from build123d import *

# Parameters (mm, degrees)
PAD_DEPTH    = 17
PAD001_DEPTH = 2
PAD002_DEPTH = 1.8
SKETCH003_W  = 32
SKETCH003_H  = 11
PAD003_DEPTH = 5
SKETCH004_W  = 3.1
SKETCH004_H  = 3.1
POCKET_DEPTH = 3.1
FILLET_R     = 3
FILLET001_R  = 1


with BuildPart() as part:
    # Sketch → Pad (new body)
    with BuildSketch(Plane.XY):
        with BuildLine():
            Line((-10, 0), (-10, 5))
            Line((-10, 5), (5, 5))
            Line((5, 5), (5, -10))
            Line((5, -10), (0, -10))
            Line((0, -7.05), (0, -10))
            Line((0, -7.05), (0.143534, -7.05))
            ThreePointArc((0.143534, -7.05), (3.05, -6.3), (0.143534, -5.55))
            Line((0, -5.55), (0.143534, -5.55))
            Line((0, 0), (0, -5.55))
            Line((0, 0), (-5.55, 0))
            Line((-5.55, 0), (-5.55, 0.143534))
            ThreePointArc((-5.55, 0.143534), (-6.3, 3.05), (-7.05, 0.143534))
            Line((-7.05, 0), (-7.05, 0.143534))
            Line((-10, 0), (-7.05, 0))
        make_face()
    extrude(amount=-PAD_DEPTH)

    # Sketch001 (on Face16 of Pad) → Pad001 (join)
    with BuildSketch(Plane(origin=(0, 0, -17), x_dir=(1, 0, 0), z_dir=(0, 0, -1))):
        Polygon((5, -5), (-10, -5), (-10, 0), (0, 10), (5, 10), align=None)
    extrude(amount=PAD001_DEPTH)

    # Sketch002 (on Face1 of Pad001) → Pad002 (join)
    with BuildSketch(Plane.XY):
        Polygon((0, -10), (0, 0), (-10, 0), align=None)
    extrude(amount=-PAD002_DEPTH)

    # Sketch003 (on Face10 of Pad002) → Pad003 (join)
    with BuildSketch(Plane.XZ):
        with Locations((-26, -13.5)):
            Rectangle(SKETCH003_W, SKETCH003_H)
    extrude(amount=-PAD003_DEPTH)

    # Sketch004 (on Face22 of Pad003) → Pocket (cut)
    with BuildSketch(Plane.XZ):
        with Locations((-36.45, -13.45)):
            Rectangle(SKETCH004_W, SKETCH004_H)
    extrude(amount=-POCKET_DEPTH, mode=Mode.SUBTRACT)

    # Fillet
    fillet_edges = [part.edges().sort_by_distance(p)[0] for p in [
        (-10, 2.5, -8),
        (-42, 2.5, -8),
        (-42, 2.5, -19),
        (-10, 0, -18),
    ]]
    fillet(fillet_edges, radius=FILLET_R)

    # Fillet001
    fillet001_edges = [part.edges().sort_by_distance(p)[0] for p in [
        (-10, 5, -2.5),
        (-10.87868, 5, -7.12132),
        (-2.5, 5, 0),
        (-26, 5, -8),
        (5, 5, -9.5),
        (-41.12132, 5, -8.87868),
        (-17, 5, -19),
        (-42, 5, -13.5),
        (-41.12132, 5, -18.12132),
        (5, -2.5, 0),
        (5, -10, -9.5),
        (5, -2.5, -19),
        (0, 0, -9.4),
    ]]
    fillet(fillet001_edges, radius=FILLET001_R)


solid = part.part
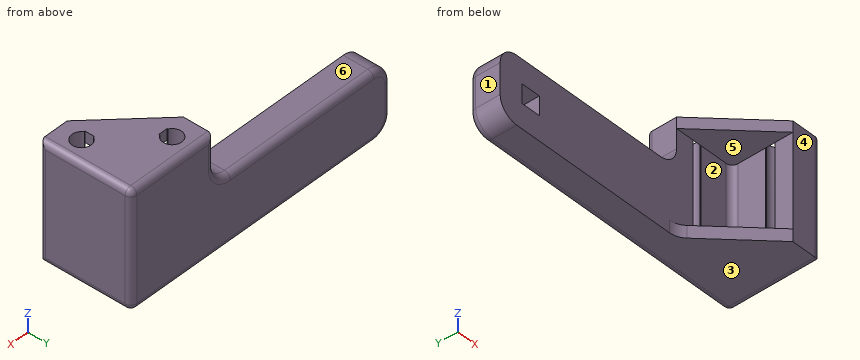
Design review of the part built by this model. Coordinates are the model's own, in mm. Face numbers are marked on the shaded views. A direction names the side the tool comes from. Round coordinates to 2 decimals unless told otherwise and drop trailing zeros. Loops run counter-clockwise (first coordinate to the right, second up) from the corner with the lowest first, then second, coordinate; pieces in that order, holes last. Notation, with made-up numbers: (20, 58) - (51, 58) arc R13 cw to (51, 82) - close; hole circle Ø8 at (52.25, -10). An arc over 180 degrees is marked (long way). One line per item, written item: value. Start each with the question number.
1) Consider section C-C on y = -4. Give the boundary of the cut face in (x, z), then the cut area to 3 significant figures.
2) Insertion check: pin 1 Ø1.5 at (x, y) = (-36.5, 2.5) entering from +Z; pin 2 Ø1.4 at (x, z) = (-3, -6.5) entering from -Y; pin 3 Ø0.9 at (y, z) = (-8.5, -10.5) entering from -X. Each pin has a flat end and moves straight along its axis. Give the tip position at first contact, or say it passes through.
3) Consider section A-A on y = 1.5. Give the boundary of the cut face in (x, z), then the cut area to 3 significant figures.
4) Draft analysis for pull direction Z (two halves, no side actions). For the marked faces 1, 2 and 3, state which applies: +Z half, -Z half, draft (parallel to the pull), parting line (faces both ways), or undercut.
5) For the marked faces 4, 5 and 6, list the 3-axis set-ups (+Z, -Z, +X, -X, +Y, -Y) from which the entire face can be reached by the end or side of a thin tool; tool diameter is ignored.
6) To check wall thickness, follow L1, parallel to X at y = -6.3, z = -10; L2, parallel to Y at x = 1.5, z = -6.5; L3, parallel to Z at x = -4.5, y = -3.5. State the ranges of each line that lie inside material, in increasing order. Write a range as from..to.
7) Consider section D-D on z = -13.25. Give the boundary of the cut face in (x, y).
8) Consider section B-B on x = -6.3. Give the boundary of the cut face in (y, z).
Reported:
1. outline: (-6, -19) - (4, -19) arc R1 ccw to (5, -18) - (5, -1) arc R1 ccw to (4, 0) - (-6, 0) - (-6, -1.8) - (0, -1.8) - (0, -17) - (-6, -17) - close
1. area: 117 mm^2
2. pin 1: stops at z = -8
2. pin 2: stops at y = 0
2. pin 3: stops at x = 0
3. outline: (-42, -16) arc R3 ccw to (-39, -19) - (4, -19) arc R1 ccw to (5, -18) - (5, -1) arc R1 ccw to (4, 0) - (-4.75, 0) - (-4.75, -17) - (-7.85, -17) - (-7.85, 0) - (-10, 0) - (-10, -5) arc R3 cw to (-13, -8) - (-39, -8) arc R3 ccw to (-42, -11) - close; hole (-38, -15) - (-34.9, -15) - (-34.9, -11.9) - (-38, -11.9) - close
3. area: 572 mm^2
4. face 1: draft
4. face 2: undercut
4. face 3: -Z half
5. face 4: +Z, -Z, +X, -X, -Y
5. face 5: -X, -Y
5. face 6: +Z, -X, +Y, -Y
6. L1: x = 3.05..5
6. L2: y = -10..-7.85, -4.75..5
6. L3: z = -19..-17, -1.8..0
7. outline: (-42, 0) - (-38, 0) - (-38, 3.1) - (-34.9, 3.1) - (-34.9, 0) - (-7.05, 0) - (-7.05, 0.14) arc R1.55 cw (long way) to (-5.55, 0.14) - (-5.55, 0) - (-1, 0) arc R1 cw to (0, -1) - (0, -5.55) - (0.14, -5.55) arc R1.55 cw (long way) to (0.14, -7.05) - (0, -7.05) - (0, -10) - (4, -10) arc R1 ccw to (5, -9) - (5, 4) arc R1 ccw to (4, 5) - (-41, 5) arc R1 ccw to (-42, 4) - close
8. outline: (-3.7, -19) - (4, -19) arc R1 ccw to (5, -18) - (5, -1) arc R1 ccw to (4, 0) - (3.05, 0) - (3.05, -17) - (-3.7, -17) - close; (-3.7, -1.8) - (0, -1.8) - (0, 0) - (-3.7, 0) - close
